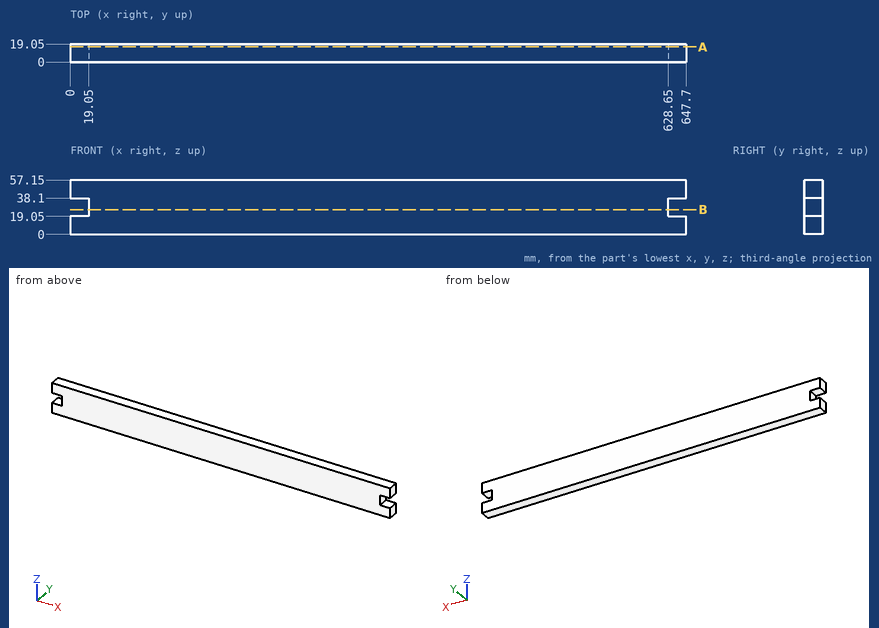
Input: dimensioned drawing with shaded views. Units: mm. Origin: part minimum x, y, z. Give positions to 0.01 mm unless a question says otherwise; leave off trailing zeros. Write each loop counter-clockwise with the first axis right and the second up, starting at its lowest first coordinate (ties: lowest second). Pieces come first, ordered by that corner, then holes. Notation, with made-up numbers: (68, -13) - (108, -13) arc R11 ccw to (108, -1) - close; hole circle Ø3 at (-18.75, 35.25). An arc over 180 degrees is marked (long way). One line per item, written item: value. Start each with the question number.
Q1. Section query B-B, the plane z = 26. Return the cut outline in (x, y).
Q2. Material intervals for probe 1 along X at (y, z) = (3, 20.5), sorted ascending. Write a range as from..to.
Q3. First-contact query: pin 1 Ø4 at (y, z) = (10.5, 29.5) entering from -X; pin 2 Ø5.5 at (y, z) = (13.5, 30) entering from +X. Flat tips, straight axial feed; report the tip coordinate or a pass-through.
Q4. Section query A-A, the plane y = 16. Return the cut outline in (x, z), then the cut area to 3 significant figures.
Answer:
1. outline: (19.05, 0) - (628.65, 0) - (628.65, 19.05) - (19.05, 19.05) - close
2. probe 1: x = 19.05..628.65
3. pin 1: stops at x = 19.05
3. pin 2: stops at x = 628.65
4. outline: (0, 0) - (647.7, 0) - (647.7, 19.05) - (628.65, 19.05) - (628.65, 38.1) - (647.7, 38.1) - (647.7, 57.15) - (0, 57.15) - (0, 38.1) - (19.05, 38.1) - (19.05, 19.05) - (0, 19.05) - close
4. area: 36,300 mm2
